Geometry check sheet. Reference: the model listing, model coordinates, mm. Round coordinates to 2 decimals unless told otherwise and drop trailing zeros. Order: outer loops, then holes, each group sorted by start corner. A loop starts at its lowest first (then second) coordinate and runs counter-clockwise, first axis right, second up. Notation, with made-up numbers: M -8,51.5 L 39,51.5 A24 ccw 39,73.5 Z; hole C -7.75,-15.75 d1. An arc over 180 degrees is marked long. Return JSON: item names as keys, results as strings. Group by question number.
```python
from build123d import *

# Parameters (mm, degrees)
F0_W     = 19
F0_H     = 19
F1_DEPTH = 16
F2_R     = 4
F3_DEPTH = 19
F4_R     = 4
F5_DEPTH = 19
F6_R     = 2


with BuildPart() as f1:
    # F0 (on Front) → F1 (new body)
    with BuildSketch(Plane.XZ):
        Rectangle(F0_W, F0_H)
    extrude(amount=F1_DEPTH)

    # F2 (on face) → F3 (cut)
    with BuildSketch(Plane.XY.offset(9.5)):
        with Locations((0, -8)):
            Circle(F2_R)
    extrude(amount=-F3_DEPTH, mode=Mode.SUBTRACT)

    # F4 (on face) → F5 (cut)
    with BuildSketch(Plane(origin=(-9.5, 0, 0), x_dir=(0, -1, 0), z_dir=(-1, 0, 0))):
        with Locations((8, 0)):
            Circle(F4_R)
    extrude(amount=-F5_DEPTH, mode=Mode.SUBTRACT)

    # F6
    f6_edges = [f1.edges().sort_by_distance(p)[0] for p in [
        (9.5, 0, 0),
        (0, 0, 9.5),
        (0, 0, -9.5),
        (-9.5, 0, 0),
        (-9.5, -16, 0),
        (9.5, -16, 0),
        (0, -16, -9.5),
        (0, -16, 9.5),
        (-9.5, -8, -9.5),
        (9.5, -8, -9.5),
        (9.5, -8, 9.5),
        (-9.5, -8, 9.5),
    ]]
    fillet(f6_edges, radius=F6_R)


solid = f1.part
```
Q1. Section check C-C on z = -6.25. Record the cut outline in (x, y), plus the area to 3 significant figures.
Q2. Section check D-D on z = 1.5. Record the cut outline in (x, y), plus the area to 3 significant figures.
Q3. Release check for a two-part mould opening along Z. For faces 1 (the face through (8.9, -0.57, 0.11)), 2 (the face through (-3, -5, 9.5)), 3 (the face through (5.7, -4.8, -2.4)) record: +Z half, -Z half, draft (parallel to the pull), parting line (faces both ways), or undercut.
Q4. Material ranges on line 1 along Y through (x, z) = (4, 0); line 2 along Z through (x, y) = (4.25, -8), recorded low to high.
Q5. Section check A-A on x = -5.5. Record the cut outline in (y, z).
Q6. Section check B-B on y = -8. Record the cut outline in (x, z), plus the area to 3 significant figures.
Q7. Depth check by flat-ended pin: pin 1 Ø5 at (y, z) = (-8, 0) entering from +X. Enter the tip coordinate at first touch or a pass-through.
Geometry check:
{
 "1": {"outline": "M -9.5,-14 A2 ccw -7.5,-16 L 7.5,-16 A2 ccw 9.5,-14 L 9.5,-2 A2 ccw 7.5,0 L -7.5,0 A2 ccw -9.5,-2 Z; hole C 0,-8 d8", "area": "250 mm^2"},
 "2": {"outline": "M -9.5,-14 A2 ccw -7.5,-16 L 7.5,-16 A2 ccw 9.5,-14 L 9.5,-11.71 L 1.5,-11.71 A4 cw -1.5,-11.71 L -9.5,-11.71 Z; M -9.5,-4.29 L -1.5,-4.29 A4 cw 1.5,-4.29 L 9.5,-4.29 L 9.5,-2 A2 ccw 7.5,0 L -7.5,0 A2 ccw -9.5,-2 Z", "area": "158 mm^2"},
 "3": {"face 1": "draft", "face 2": "+Z half", "face 3": "undercut"},
 "4": {"line 1": "y = -16 to -12, -4 to 0", "line 2": "z = -9.5 to -4, 4 to 9.5"},
 "5": {"outline": "M -16,-7.5 A2 ccw -14,-9.5 L -2,-9.5 A2 ccw 0,-7.5 L 0,7.5 A2 ccw -2,9.5 L -14,9.5 A2 ccw -16,7.5 Z; hole C -8,0 d8"},
 "6": {"outline": "M -9.5,-7.5 A2 ccw -7.5,-9.5 L -4,-9.5 L -4,-4 L -9.5,-4 Z; M -9.5,4 L -4,4 L -4,9.5 L -7.5,9.5 A2 ccw -9.5,7.5 Z; M 4,-9.5 L 7.5,-9.5 A2 ccw 9.5,-7.5 L 9.5,-4 L 4,-4 Z; M 4,4 L 9.5,4 L 9.5,7.5 A2 ccw 7.5,9.5 L 4,9.5 Z", "area": "118 mm^2"},
 "7": {"pin 1": "passes through"}
}
